Verification items for the finished model (mm, model axes). Coordinates: 2 decimals unless noted, no trailing zeros. Order: outer loops, then holes, each group sorted by start corner. A loop starts at its lowest first (then second) coordinate and runs counter-clockwise, first axis right, second up. Notation, with made-up numbers: (83.5, 34) -> (124.5, 34) arc R14 cw to (124.5, 52) -> close; hole circle Ø11 at (88, 1). An arc over 180 degrees is marked (long way). Write each question's results on one line, items separated by ' | '. Start each with the question number.
(1) Go/stop test with flat-tipped pins: pin 1 (1.5 mm diameter, centred on x = -845, z = 0.5, fed in from -Y); pin 2 (2.5 mm diameter, centred on x = -890, z = -1, fed in from +Y). Record where each tip stops, or that it passes through.
(2) Cross-section at A-A on x = -844.5. Enter the section's corners in (y, z), and give its area (3 significant figures).
(3) Cross-section at B-B on y = -58.5. Enter the section's corners in (x, z), and give its area (4 significant figures).
(4) Thickness scan on probe 1 along X at (y, z) = (-148, 1); probe 2 along Y at (x, z) = (-857, -2.15); probe 3 along X at (y, z) = (-87.5, -0.4). Record the ranges inside material, lowest first. Write a range as [from, to].
```python
from build123d import *

# Parameters (mm, degrees)
BOSS_EXTRUDE1_DEPTH = 2.5


with BuildPart() as part:
    # Sketch2 → Boss-Extrude1 (new, symmetric)
    with BuildSketch(Plane.XY):
        Polygon((-936.252975542, -80.979102057), (-936.252975542, -13.729117514), (-891.502975542, -13.729117514), (-891.502975542, -23.979117514), (-886.002975542, -23.979117514), (-886.002975542, -13.729117514), (-846.502975542, -13.729117514), (-846.502975542, -23.979117514), (-841.002975542, -23.979117514), (-841.002975542, -13.729117514), (-796.252975542, -13.729117514), (-796.252975542, -80.979102057), (-806.502975542, -80.979102057), (-806.502975542, -86.479102057), (-796.252975542, -86.479102057), (-796.252975542, -153.729086599), (-841.002975542, -153.729086599), (-841.002975542, -143.479086599), (-846.502975542, -143.479086599), (-846.502975542, -153.729086599), (-886.002975542, -153.729086599), (-886.002975542, -143.479086599), (-891.502975542, -143.479086599), (-891.502975542, -153.729086599), (-936.252975542, -153.729086599), (-936.252975542, -86.479102057), (-926.002975542, -86.479102057), (-926.002975542, -80.979102057), align=None)
        Polygon((-881.252975542, -43.479117514), (-881.252975542, -48.729117514), (-851.252975542, -48.729117514), (-851.252975542, -43.479117514), (-826.002975542, -43.479117514), (-826.002975542, -63.979117514), (-831.252975542, -63.979117514), (-831.252975542, -103.479086599), (-826.002975542, -103.479086599), (-826.002975542, -123.979086599), (-851.252975542, -123.979086599), (-851.252975542, -118.729086599), (-881.252975542, -118.729086599), (-881.252975542, -123.979086599), (-906.502975542, -123.979086599), (-906.502975542, -103.479086599), (-901.252975542, -103.479086599), (-901.252975542, -63.979117514), (-906.502975542, -63.979117514), (-906.502975542, -43.479117514), align=None, mode=Mode.SUBTRACT)
    extrude(amount=BOSS_EXTRUDE1_DEPTH, both=True)


solid = part.part
```
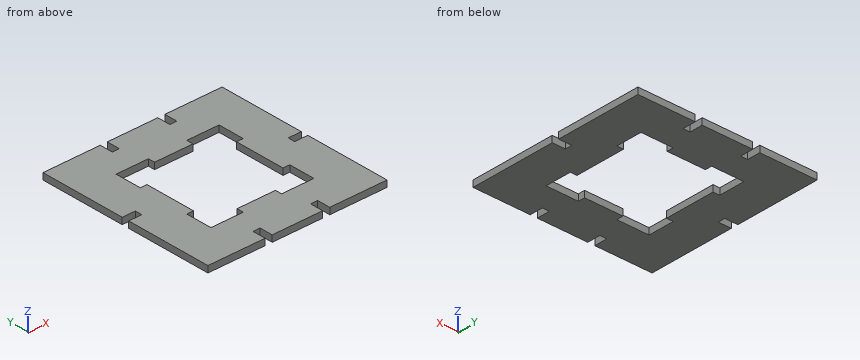
Results are:
1) pin 1: stops at y = -143.48 | pin 2: stops at y = -23.98
2) outline: (-143.48, -2.5) -> (-123.98, -2.5) -> (-123.98, 2.5) -> (-143.48, 2.5) -> close; (-43.48, -2.5) -> (-23.98, -2.5) -> (-23.98, 2.5) -> (-43.48, 2.5) -> close | area: 195 mm2
3) outline: (-936.25, -2.5) -> (-906.5, -2.5) -> (-906.5, 2.5) -> (-936.25, 2.5) -> close; (-826, -2.5) -> (-796.25, -2.5) -> (-796.25, 2.5) -> (-826, 2.5) -> close | area: 297.5 mm2
4) probe 1: x = [-936.25, -891.5], [-886, -846.5], [-841, -796.25] | probe 2: y = [-153.73, -118.73], [-48.73, -13.73] | probe 3: x = [-936.25, -901.25], [-831.25, -796.25]
